from build123d import *

# Parameters (mm, degrees)
EXTRUDE_1_DEPTH     = 15
SKETCH_2_R          = 6.260668565
CUT_EXTRUDE_1_DEPTH = 20
SKETCH_3_R          = 2
CUT_EXTRUDE_2_DEPTH = 20


with BuildPart() as part:
    # 草图1 → 凸台-拉伸1 (new body)
    with BuildSketch(Plane.XY):
        Polygon((-10.368613139, -4.854014599), (9.631386861, -4.854014599), (8.131386861, 0), (3.131386861, 0), (3.131386861, 12.518248175), (-3.868613139, 12.518248175), (-3.868613139, 0), (-8.868613139, 0), align=None)
    extrude(amount=EXTRUDE_1_DEPTH)

    # 草图2 → 切除-拉伸1 (cut)
    with BuildSketch(Plane(origin=(3.131386861, 0, 0), x_dir=(0, 0, -1), z_dir=(1, 0, 0))):
        with Locations((-7.5, 6.259124088)):
            Circle(SKETCH_2_R)
    extrude(amount=-CUT_EXTRUDE_1_DEPTH, mode=Mode.SUBTRACT)

    # 草图3 → 切除-拉伸2 (cut)
    with BuildSketch(Plane.XZ.offset(4.854014599)):
        with Locations(Location((-7.868613139, 12.5, 0), (0, 0, 270))):
            Circle(SKETCH_3_R)
        with Locations(Location((7.131386861, 12.5, 0), (0, 0, 270))):
            Circle(SKETCH_3_R)
        with Locations(Location((7.131386861, 2.5, 0), (0, 0, 270))):
            Circle(SKETCH_3_R)
        with Locations(Location((-7.868613139, 2.5, 0), (0, 0, 270))):
            Circle(SKETCH_3_R)
    extrude(amount=-CUT_EXTRUDE_2_DEPTH, mode=Mode.SUBTRACT)


solid = part.part
Work out the finished part from the listing and answer in its coordinate system (mm). A direction names the side the tool comes from. Round coordinates to 2 decimals unless told otherwise and drop trailing zeros. Order: outer loops, then holes, each group sorted by start corner. A loop starts at its lowest first (then second) coordinate and runs counter-clockwise, first axis right, second up. Notation, with made-up numbers: M 82,-33 L 116,-33 A34 ccw 116,3 Z; hole C -27.5,53 d11. An arc over 180 degrees is marked long. Put each result on its own line as item: value. Start each with the question number.
Q1. Straight lines are drawn through the part: L1, parallel to X at y = 9.75, z = 0.5; L2, parallel to X at y = -2.2, z = 12.5; L3, parallel to Y at x = 6.5, z = 8.5. For each, find the intervals that lie inside material, in ascending order. Write a range as [from, to].
Q2. Section A-A, the plane y = 6.75 is taken. Write down the section's boundary in (x, z), and give its area (3 significant figures).
Q3. Section C-C, the plane x = -7.5 is taken. Write down the section's boundary in (y, z), and give its area (3 significant figures).
Q4. For a pull along X with two mould halves and no side action, classify faces 1 (the flat face through (8.89, -2.46, 7.4)), 2 (the cylindrical face through (5.18, -2.46, 12.93)), 3 (the flat face through (-3.869, 7, 14)) as pulls with the +X half, pulls with the -X half, needs draft (parallel to the pull), parting line crosses it, or undercut.
Q5. A tool of negligible diameter and unlimited length cuts with its end or side. For faces 4 (the cylindrical face through (-0.118, 0.004, 7.773)), 5 (the flat face through (3.131, 7, 1)), 6 (the flat face through (-3.869, 6, 1)), from which of +Z, -Z, +X, -X, +Y, -Y can it reach the whole face along a straight path? Write none if from no direction.
Q6. Section B-B, the plane z = 5.25 is taken. Write down the section's boundary in (x, y), and give its area (3 significant figures).
Q7. Section D-D, the plane z = 12.5 is taken. Write down the section's boundary in (x, y), and give its area (3 significant figures).
Q8. Flat-ended cylindrical pins translate along their axes: pin 1 (3 mm diameter, centred on x = -7.87, z = 12.5, fed in from -Y); pin 2 (4 mm diameter, centred on x = -6, z = 12, fed in from +Y); pin 3 (8 mm diameter, centred on y = 6.5, z = 4.5, fed in from +X); pin 4 (6 mm diameter, centred on y = 8, z = 11.5, fed in from -X). Find the tip coordinate at first contact, or state that the pin passes through.
Findings below:
1. L1: x = [-3.87, 3.13]
1. L2: x = [-5.87, 5.13]
1. L3: y = [-4.85, 0]
2. outline: M -3.87,0 L 3.13,0 L 3.13,1.26 L -3.87,1.26 Z; M -3.87,13.74 L 3.13,13.74 L 3.13,15 L -3.87,15 Z
2. area: 17.6 mm^2
3. outline: M -4.85,0 L 0,0 L 0,0.53 L -4.85,0.53 Z; M -4.85,4.47 L 0,4.47 L 0,7.36 A6.26 cw 0,7.64 L 0,10.53 L -4.85,10.53 Z; M -4.85,14.47 L 0,14.47 L 0,15 L -4.85,15 Z
3. area: 34.6 mm^2
4. face 1: pulls with the +X half
4. face 2: undercut
4. face 3: pulls with the -X half
5. face 4: +X, -X
5. face 5: +Z, -Z, +X, +Y
5. face 6: +Z, -Z, -X, +Y
6. outline: M -10.37,-4.85 L 9.63,-4.85 L 8.13,0 L 3.13,0 L 3.13,0.42 L -3.87,0.42 L -3.87,0 L -8.87,0 Z; M -3.87,12.1 L 3.13,12.1 L 3.13,12.52 L -3.87,12.52 Z
6. area: 95.6 mm^2
7. outline: M -10.37,-4.85 L -9.87,-4.85 L -9.87,-3.24 Z; M -5.87,-4.85 L 5.13,-4.85 L 5.13,0 L 3.13,0 L 3.13,2.49 L -3.87,2.49 L -3.87,0 L -5.87,0 Z; M -3.87,10.03 L 3.13,10.03 L 3.13,12.52 L -3.87,12.52 Z; M 9.13,-4.85 L 9.63,-4.85 L 9.13,-3.24 Z
7. area: 89.1 mm^2
8. pin 1: passes through
8. pin 2: stops at y = 0
8. pin 3: stops at x = 3.13
8. pin 4: stops at x = -3.87
